```python
from build123d import *

# Parameters (mm, degrees)
BASEHEAD_DEPTH  = 8.2042
SKETCH4_W       = 0.381
SKETCH4_H       = 27.119109733
HEADFILLET_R    = 0.381
THDSCHPAT_COUNT = 17
THDSCHPAT_PITCH = 1.867647059


with BuildPart() as part:
    # Sketch1 → BaseHead (new body)
    with BuildSketch(Plane(origin=(0, 0, 0), x_dir=(0, 0, -1), z_dir=(1, 0, 0))):
        Polygon((11.1125, 6.415804866), (11.1125, -6.415804866), (0, -12.831609733), (-11.1125, -6.415804866), (-11.1125, 6.415804866), (0, 12.831609733), align=None)
    extrude(amount=BASEHEAD_DEPTH)

    # BodySke → BaseBody (revolve)
    with BuildSketch(Plane.XY, mode=Mode.PRIVATE) as basebody_sk:
        Polygon((0, 0), (109.8042, 0), (109.8042, 5.18668), (108.64088, 6.35), (0, 6.35), align=None)
    revolve(basebody_sk.sketch.rotate(Axis((0, 0, 0), (1, 0, 0)), 90), axis=Axis((0, 0, 0), (1, 0, 0)))

    # Sketch3 → HeadChamfer (revolve, cut)
    with BuildSketch(Plane.XY):
        Polygon((0, 11.1125), (4.658702676, 19.181609733), (4.658702676, 25.531609733), (-12.7, 25.531609733), (-12.7, 11.1125), align=None)
    revolve(axis=Axis((0, 0, 0), (1, 0, 0)), mode=Mode.SUBTRACT)

    # Sketch4 → BearingFace (revolve, cut)
    with BuildSketch(Plane.XY, mode=Mode.PRIVATE) as bearingface_sk:
        with Locations((8.0137, 24.672054866)):
            Rectangle(SKETCH4_W, SKETCH4_H)
    revolve(bearingface_sk.sketch.rotate(Axis((0, 0, 0), (1, 0, 0)), 270), axis=Axis((0, 0, 0), (1, 0, 0)), mode=Mode.SUBTRACT)

    # HeadFillet
    headfillet_edges = [part.edges().sort_by_distance(p)[0] for p in [
        (8.2042, 0, -6.35),
    ]]
    fillet(headfillet_edges, radius=HEADFILLET_R)

    # ThdSchSke → ThreadSchematic (revolve, cut)
    with BuildSketch(Plane.XY):
        Polygon((78.0542, -5.18668), (77.239634567, -6.35), (77.239634567, -7.9375), (78.868765433, -7.9375), (78.868765433, -6.35), align=None)
    threadschematic = revolve(axis=Axis((-3.175, 0, 0), (1, 0, 0)), mode=Mode.SUBTRACT)

    # ThdSchPat: ThreadSchematic ×17
    with Locations(*[(i * THDSCHPAT_PITCH, 0, 0) for i in range(1, THDSCHPAT_COUNT)]):
        add(threadschematic, mode=Mode.SUBTRACT)


solid = part.part
```
Could you check a few things on this model? Use its own coordinates, in mm. A direction names the side the tool comes from. Round coordinates to 2 decimals unless told otherwise and drop trailing zeros. Loops run counter-clockwise (first coordinate to the right, second up) from the corner with the lowest first, then second, coordinate; pieces in that order, holes last. Notation, with made-up numbers: M 5,-31 L 41,-31 A19 cw 41,-6 Z; hole C 44,-39 d2. An arc over 180 degrees is marked long. Put each result on its own line as item: value.
Q1. For pin 1 (4.5 mm diameter, centred on y = 4, z = -9.5, fed in from +X); pin 2 (3 mm diameter, centred on x = 61.5, z = -4, fed in from -Y); pin 3 (5 mm diameter, centred on x = 22, z = 1, fed in from -Y), each with a flat end and sliding along its axis, tell me the tip position at first contact or that it passes through.
Check result:
pin 1: x = 8.2
pin 2: y = -5.84
pin 3: y = -6.35
Q2. I need wall thicknesses on probe 1 along X at (y, z) = (-7.75, 3); probe 2 along Z at (x, y) = (101.5, -0.25); probe 3 along Y at (x, z) = (7, -3). Which ranges of each line are inside material? Lowest first, please.
Check result:
probe 1: 0 to 8.2
probe 2: -6.35 to 6.35
probe 3: -11.1 to 11.1
Q3. Imagine slicing it at A-A (x = 26.5). Write out the boundary of the cut face in (y, z).
Check result:
outline: C 0,0 d12.7
Q4. On a 3-axis mill with a long thin cutter (end or side, diameter ignored), from which of +Z, -Z, +X, -X, +Y, -Y can I reach the whole of each face in a straight line? I mean faces 1 (the face through (8.204, -5, 5)), 2 (the face through (109.804, 0, 0)). Say none if no direction works.
Check result:
face 1: +X
face 2: +Z, -Z, +X, +Y, -Y
